The model under review builds one solid part; all positions refer to its coordinate system, in mm. Round coordinates to 2 decimals unless told otherwise and drop trailing zeros. Loops run counter-clockwise (first coordinate to the right, second up) from the corner with the lowest first, then second, coordinate; pieces in that order, holes last. Notation, with made-up numbers: (47.5, -2.75) -> (81.5, -2.75) arc R31 cw to (81.5, 23.25) -> close; hole circle Ø7 at (-40, 82.5). An arc over 180 degrees is marked (long way). Return JSON: item names as keys, results as strings. Group by question number.
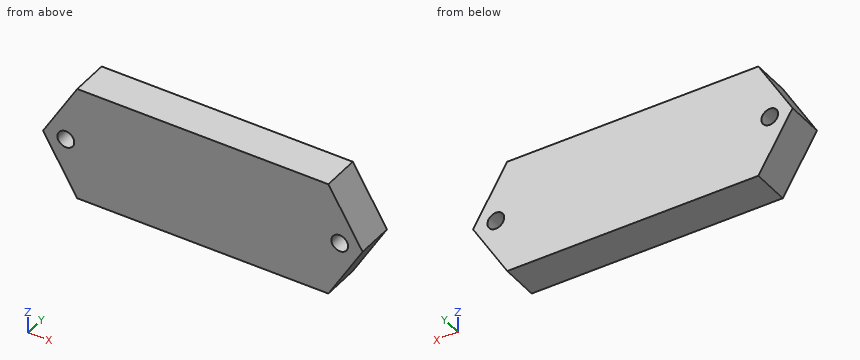
```python
from build123d import *

# Parameters (mm, degrees)
SKETCH_1_W      = 33
SKETCH_1_H      = 15
SKETCH_1_R      = 1.1
EXTRUDE_1_DEPTH = 5


with BuildPart() as part:
    # 草图1 → 凸台-拉伸1 (new body)
    # profile 1 of 3: a face of its own
    with BuildSketch(Plane(origin=(0, 0, 0), x_dir=(1, 0, 0), z_dir=(0, 1, 0))):
        Rectangle(SKETCH_1_W, SKETCH_1_H)
    # profile 2 of 3: a face of its own
    with BuildSketch(Plane(origin=(0, 0, 0), x_dir=(1, 0, 0), z_dir=(0, 1, 0))):
        Polygon((-21, 0), (-16.5, 7.5), (-16.5, -7.5), align=None)
        with Locations(Location((-18, 0, 0), (0, 0, 270))):
            Circle(SKETCH_1_R, mode=Mode.SUBTRACT)
    # profile 3 of 3: a face of its own
    with BuildSketch(Plane(origin=(0, 0, 0), x_dir=(1, 0, 0), z_dir=(0, 1, 0))):
        Polygon((16.5, 7.5), (16.5, -7.5), (21, 0), align=None)
        with Locations(Location((18, 0, 0), (0, 0, 270))):
            Circle(SKETCH_1_R, mode=Mode.SUBTRACT)
    extrude(amount=EXTRUDE_1_DEPTH)


solid = part.part
```
1. Wall thickness on line 1 (X direction, y = 3.6, z = -1); line 2 (Z direction, x = -17, y = 0.55); line 3 (X direction, y = 1.3, z = 7): over which ranges is each line inside the solid? List them lowest first.
2. We need section D-D, the plane z = -1.75. Write out the cut boundary in (x, y).
3. We need section B-B, the plane x = -18. Write out the cut boundary in (y, z), then the cut area to 3 significant figures.
4. We need section C-C, the plane z = 2.25. Write out the cut boundary in (x, y).
5. For P1, Ø3, axis at y = 3, z = -4.5, coming from the +X side; P2, Ø1.3, axis at x = 18, z = 0, coming from the -Y side; P3, Ø1.5, axis at y = 3.5, z = 5.5, coming from the +X side, all flat-tipped, find the tip position at first contact; note any pin that passes through.
6. We need section A-A, the plane y = 2.3. Write out the cut boundary in (x, z).
Check sheet entries:
{
 "1": {"line 1": "x = -20.4 to -18.46, -17.54 to 17.54, 18.46 to 20.4", "line 2": "z = -6.67 to -0.46, 0.46 to 6.67", "line 3": "x = -16.8 to 16.8"},
 "2": {"outline": "(-19.95, 0) -> (19.95, 0) -> (19.95, 5) -> (-19.95, 5) -> close"},
 "3": {"outline": "(0, -5) -> (5, -5) -> (5, -1.1) -> (0, -1.1) -> close; (0, 1.1) -> (5, 1.1) -> (5, 5) -> (0, 5) -> close", "area": "39.0 mm²"},
 "4": {"outline": "(-19.65, 0) -> (19.65, 0) -> (19.65, 5) -> (-19.65, 5) -> close"},
 "5": {"P1": "stops at x = 19.2", "P2": "passes through", "P3": "stops at x = 18.15"},
 "6": {"outline": "(-21, 0) -> (-16.5, -7.5) -> (16.5, -7.5) -> (21, 0) -> (16.5, 7.5) -> (-16.5, 7.5) -> close; hole circle Ø2.2 at (-18, 0); hole circle Ø2.2 at (18, 0)"}
}
